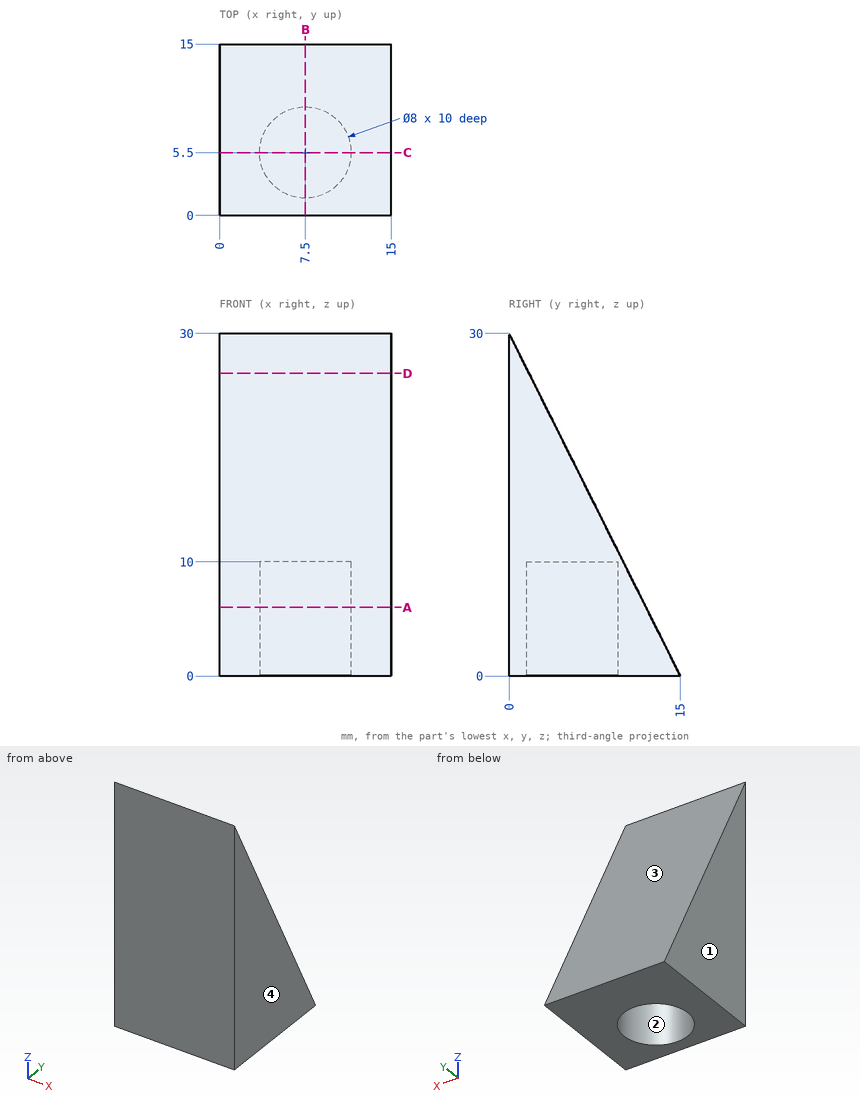
Verification items for this drawing (mm, ordinates from the low corner). Give positions to 0.01 mm unless a question says otherwise; leave off trailing zeros. Order: outer loops, then holes, each group sorted by start corner. A loop starts at its lowest first (then second) coordinate and runs counter-clockwise, first axis right, second up. Notation, with made-up numbers: M 23.5,51 L 31.5,51 A26 cw 31.5,73 Z; hole C 0,64 d6. An arc over 180 degrees is marked long. Use a Markdown table: item, result.
Item 1: Section check C-C (y = 5.5). Record the cut outline in (x, z), and give its area (3 significant figures).
Answers follow:
| item | result |
|---|---|
| outline | M 0,0 L 3.5,0 L 3.5,10 L 11.5,10 L 11.5,0 L 15,0 L 15,19 L 0,19 Z |
| area | 205 mm2 |
Item 2: Section check B-B (x = 7.5). Record the cut outline in (y, z), and give its area (3 significant figures).
Answers follow:
| item | result |
|---|---|
| outline | M 0,0 L 1.5,0 L 1.5,10 L 9.5,10 L 9.5,0 L 15,0 L 0,30 Z |
| area | 145 mm2 |
Item 3: Section check A-A (z = 6). Record the cut outline in (x, y), and give its area (3 significant figures).
Answers follow:
| item | result |
|---|---|
| outline | M 0,0 L 15,0 L 15,12 L 0,12 Z; hole C 7.5,5.5 d8 |
| area | 130 mm2 |
Item 4: Draft check along X on the marked faces 1, 2, 3 and 4. Enter one of: +X half, -X half, draft (parallel to the pull), parting line (faces both ways), or undercut.
Answers follow:
| item | result |
|---|---|
| face 1 | -X half |
| face 2 | undercut |
| face 3 | draft |
| face 4 | +X half |
Item 5: Section check D-D (z = 26.5). Record the cut outline in (x, y).
Answers follow:
| item | result |
|---|---|
| outline | M 0,0 L 15,0 L 15,1.75 L 0,1.75 Z |
Item 6: Depth check by flat-ended pin: P1, Ø4, axis at x = 7.5, y = 6.5, coming from the -Z side; P2, Ø7, axis at x = 7.5, y = 5.5, coming from the +Z side; P3, Ø3, axis at y = 7, z = 20.5, coming from the -X side; P4, Ø3, axis at x = 2, y = 8, coming from the +Z side. Enter the tip coordinate at first touch or a pass-through.
Answers follow:
| item | result |
|---|---|
| P1 | stops at z = 10 |
| P2 | stops at z = 26 |
| P3 | passes through |
| P4 | stops at z = 17 |
Item 7: Material ranges on line 1 along Y through (x, z) = (7.5, 7); line 2 along Y through (x, z) = (8.5, 23); line 3 along Y through (x, z) = (8.5, 7.5), recorded low to high.
Answers follow:
| item | result |
|---|---|
| line 1 | y = 0 to 1.5, 9.5 to 11.5 |
| line 2 | y = 0 to 3.5 |
| line 3 | y = 0 to 1.63, 9.37 to 11.25 |
